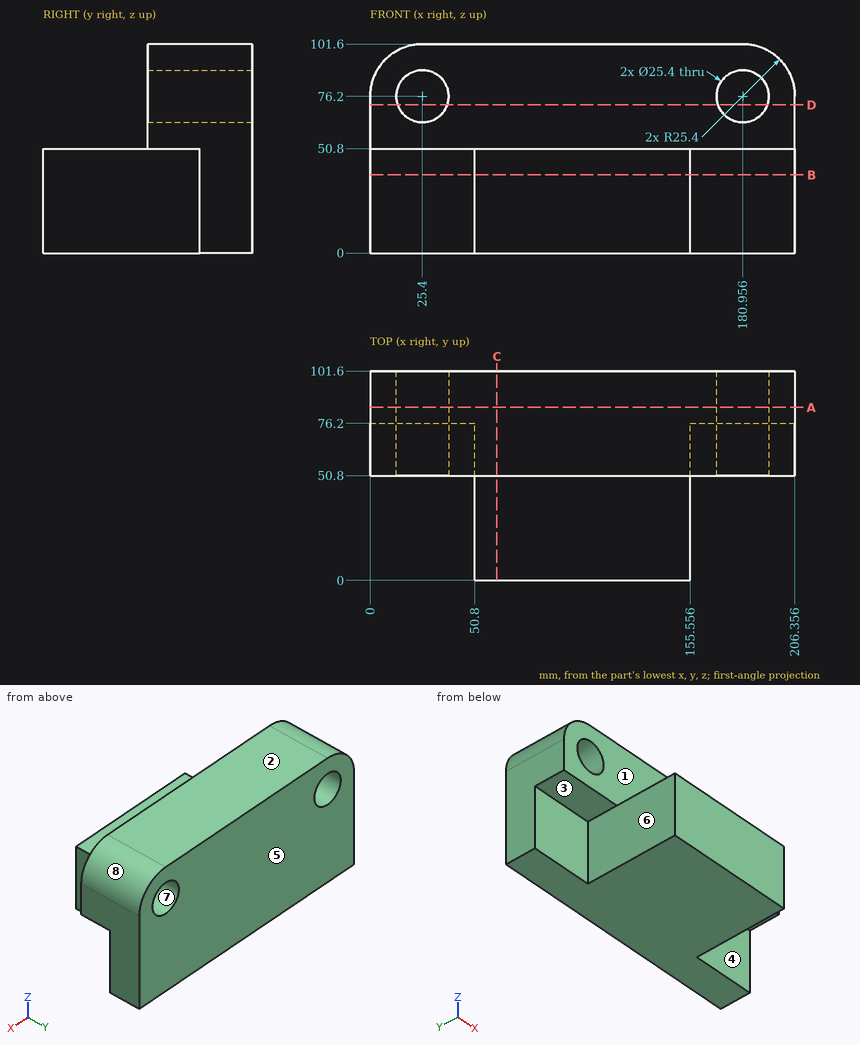
Can you work these out from the drawing? Everything is in mm from the part's minimum corner. A direction names the side the tool comes from. Give positions to 0.01 mm unless a question says otherwise; leave off trailing zeros. Order: outer loops, then holes, each group sorted by start corner. A loop starts at its lowest first (then second) coordinate and runs counter-clockwise, first axis right, second up. Notation, with made-up numbers: M -4,51.25 L 45,51.25 A31 ccw 45,85.25 Z; hole C 53.25,-9 d8. An arc over 180 degrees is marked long. Use a Markdown table: item, result. Add a question column.
1. On a 3-axis mill with a long thin cutter (end or side, diameter ignored), from which of +Z, -Z, +X, -X, +Y, -Y can I reach the whole of each face in a straight line? I mean the marked faces 1, 2, 3, 4 and 5. Say none if no direction works.
2. If we mould it in two halves opening along Z, with no side actions, what happens to the marked faces 6, 7 and 8? For each: +Z half, -Z half, draft (parallel to the pull), parting line (faces both ways), or undercut.
3. Suppose I cut it at A-A (y = 84). List the corners of the cut face in (x, z) for me.
4. For pin 1 Ø1.5 at (x, z) = (93.5, 87.5) entering from -Y; pin 2 Ø20.5 at (x, y) = (169.5, 58) entering from -Z; pin 3 Ø5 at (y, z) = (50, 24) entering from +X, each with a flat end and sliding along its axis, tell me the tip position at first contact or that it passes through.
5. Suppose I cut it at C-C (x = 61.5). List the corners of the cut face in (y, z) for me, and give its area (3 significant figures).
6. Suppose I cut it at B-B (z = 38). List the corners of the cut face in (x, y) for me.
7. I need wall thicknesses on probe 1 along X at (y, z) = (67, 76) (1 decimal); probe 2 along Y at (x, z) = (98.5, 97.5); probe 3 along X at (y, z) = (51, 27). Which ranges of each line are inside material? Lowest first, please. Write a range as from..to.
8. Suppose I cut it at D-D (z = 72). List the corners of the cut face in (x, y) for me (1 decimal).
Results list:
| question | item | result |
|---|---|---|
| 1 | face 1 | +Z, +X, -X, -Y |
| 1 | face 2 | +Z, +X, -X, +Y, -Y |
| 1 | face 3 | -Z, -X, -Y |
| 1 | face 4 | -Z, +X, -Y |
| 1 | face 5 | +Z, -Z, +X, -X, +Y |
| 2 | face 6 | draft |
| 2 | face 7 | undercut |
| 2 | face 8 | +Z half |
| 3 | outline | M 0,0 L 206.36,0 L 206.36,76.2 A25.4 ccw 180.96,101.6 L 25.4,101.6 A25.4 ccw 0,76.2 Z; hole C 25.4,76.2 d25.4; hole C 180.96,76.2 d25.4 |
| 4 | pin 1 | stops at y = 50.8 |
| 4 | pin 2 | stops at z = 50.8 |
| 4 | pin 3 | stops at x = 155.56 |
| 5 | outline | M 0,0 L 101.6,0 L 101.6,101.6 L 50.8,101.6 L 50.8,50.8 L 0,50.8 Z |
| 5 | area | 7,740 mm² |
| 6 | outline | M 0,76.2 L 50.8,76.2 L 50.8,0 L 155.56,0 L 155.56,76.2 L 206.36,76.2 L 206.36,101.6 L 0,101.6 Z |
| 7 | probe 1 | x = 0..12.7, 38.1..168.3, 193.7..206.4 |
| 7 | probe 2 | y = 50.8..101.6 |
| 7 | probe 3 | x = 50.8..155.56 |
| 8 | outline | M 0,50.8 L 13.4,50.8 L 13.4,101.6 L 0,101.6 Z; M 37.4,50.8 L 169,50.8 L 169,101.6 L 37.4,101.6 Z; M 192.9,50.8 L 206.4,50.8 L 206.4,101.6 L 192.9,101.6 Z |
